Input: dimensioned drawing with shaded views. Units: mm. Origin: part minimum x, y, z. Give positions to 0.01 mm unless a question says otherwise; leave off trailing zeros. Write each loop counter-clockwise with the first axis right and the second up, starting at its lowest first coordinate (ties: lowest second). Pieces come first, ordered by that corner, then holes. Notation, with made-up numbers: (58, 49) - (73, 49) arc R17 cw to (73, 67) - close; hole circle Ø10 at (73, 25.5). An arc over 180 degrees is marked (long way). Answer as CSV lines item,"result".
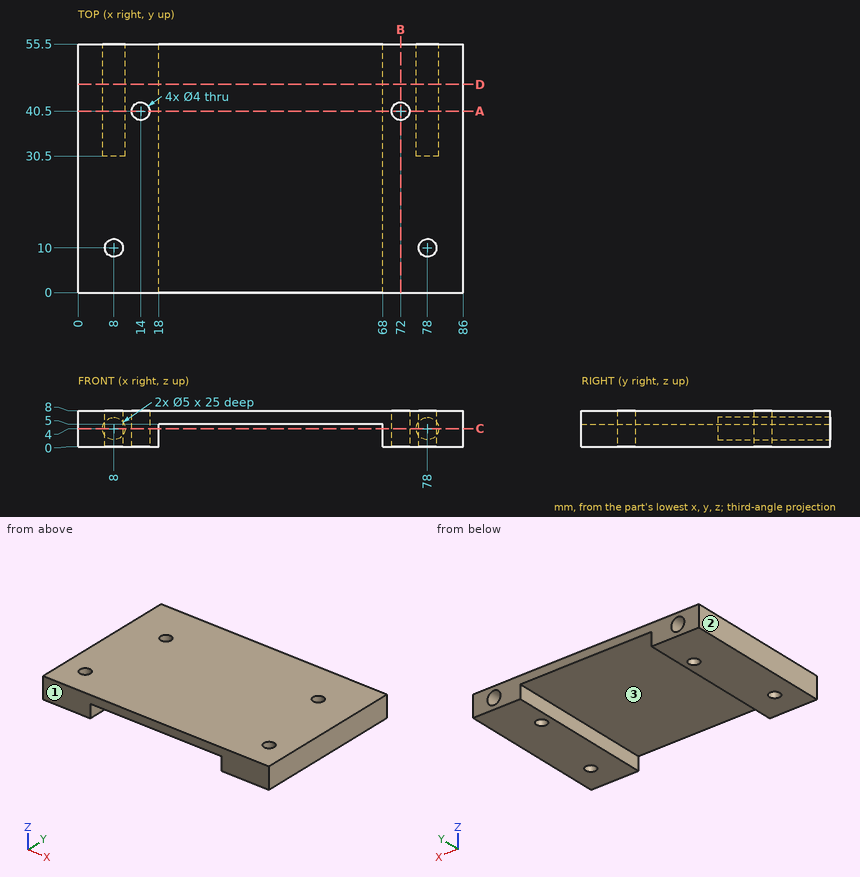
Item 1: Ray query, line 1 (X direction, y = 47.5, z = 4); line 2 (Y direction, x = 72, z = 2); line 3 (Y direction, x = 8, z = 3.75). Return the intervals inside material, ascending. Write a range as from..to.
The answers:
line 1,"0..5.5, 10.5..18, 68..75.5, 80.5..86"
line 2,"0..38.5, 42.5..55.5"
line 3,"0..8, 12..30.5"
Item 2: Cut plane A-A on y = 40.5. Return the cut outline in (x, z), plus the area to 3 significant figures.
The answers:
outline,"(0, 0) - (12, 0) - (12, 8) - (0, 8) - close; (16, 0) - (18, 0) - (18, 5) - (68, 5) - (68, 0) - (70, 0) - (70, 8) - (16, 8) - close; (74, 0) - (86, 0) - (86, 8) - (74, 8) - close; hole circle Ø5 at (8, 4); hole circle Ø5 at (78, 4)"
area,"335 mm²"
Item 3: Contact query for flat-ended pins moving along their axis: pin 1 (8 mm diameter, centred on x = 70, y = 44.5, fed in from -Z); pin 2 (25 mm diameter, centred on x = 49.5, y = 24, fed in from -Z); pin 3 (2.5 mm diameter, centred on x = 78.5, z = 4.5, fed in from +Y). Output: stop coordinate, or through.
The answers:
pin 1,"z = 0"
pin 2,"z = 5"
pin 3,"y = 30.5"
Item 4: Cut plane D-D on y = 46.5. Return the cut outline in (x, z).
The answers:
outline,"(0, 0) - (18, 0) - (18, 5) - (68, 5) - (68, 0) - (86, 0) - (86, 8) - (0, 8) - close; hole circle Ø5 at (8, 4); hole circle Ø5 at (78, 4)"
Item 5: Mould query, pull axis X, two halves, no side actions, for the marked faces 1, 2 and 3. Classes: +X half, -X half, draft (parallel to the pull), parting line (faces both ways), or undercut.
The answers:
face 1,"draft"
face 2,"-X half"
face 3,"undercut"
Item 6: Cut plane C-C on z = 4. Return the cut outline in (x, y).
The answers:
outline,"(0, 0) - (18, 0) - (18, 55.5) - (10.5, 55.5) - (10.5, 30.5) - (5.5, 30.5) - (5.5, 55.5) - (0, 55.5) - close; (68, 0) - (86, 0) - (86, 55.5) - (80.5, 55.5) - (80.5, 30.5) - (75.5, 30.5) - (75.5, 55.5) - (68, 55.5) - close; hole circle Ø4 at (8, 10); hole circle Ø4 at (14, 40.5); hole circle Ø4 at (72, 40.5); hole circle Ø4 at (78, 10)"
Item 7: Cut plane B-B on x = 72. Return the cut outline in (y, z).
The answers:
outline,"(0, 0) - (38.5, 0) - (38.5, 8) - (0, 8) - close; (42.5, 0) - (55.5, 0) - (55.5, 8) - (42.5, 8) - close"
